Model file for the job. Use its own axes, mm. Face numbers are marked on the shaded views. A direction names the side the tool comes from. Round coordinates to 2 decimals unless told otherwise and drop trailing zeros. Order: outer loops, then holes, each group sorted by start corner. A loop starts at its lowest first (then second) coordinate and runs counter-clockwise, first axis right, second up. Notation, with made-up numbers: (58.25, 15) - (106.25, 15) arc R21 ccw to (106.25, 39) - close; hole circle Ø11 at (40.25, 70.25). An arc over 180 degrees is marked (long way). Write item = value, one per line.
```python
from build123d import *

# Parameters (mm, degrees)
F0_R          = 12.7
F1_DEPTH      = 76.2
F2_DEPTH      = 79.375
F2_DEPTH_BACK = 3.175
F4_DEPTH      = 50.8
F6_DEPTH      = 50.8


with BuildPart() as f1:
    # F0 (on Front) → F1 (new body)
    with BuildSketch(Plane.XZ):
        Circle(F0_R)
        Polygon((3.6661742094, 6.35), (5.499261351, 3.174999936), (7.3323484187, 0), (5.4992613448, -3.1749999467), (3.6661742094, -6.35), (0, -6.35), (-3.6661742094, -6.35), (-5.4992613166, -3.1749999956), (-7.3323484187, 0), (-5.4992612953, 3.1750000324), (-3.6661742094, 6.35), (0, 6.35), align=None, mode=Mode.SUBTRACT)
        with BuildLine():
            ThreePointArc((0, 6.35), (3.175000032, 5.4992612955), (5.499261351, 3.174999936))
            Line((5.499261351, 3.174999936), (3.6661742094, 6.35))
            Line((3.6661742094, 6.35), (0, 6.35))
        make_face()
        with BuildLine():
            ThreePointArc((5.499261351, 3.174999936), (6.1336290065, 1.6435009007), (6.35, 0))
            ThreePointArc((6.35, 0), (6.1336290049, -1.6435009067), (5.4992613448, -3.1749999467))
            Line((5.4992613448, -3.1749999467), (7.3323484187, 0))
            Line((7.3323484187, 0), (5.499261351, 3.174999936))
        make_face()
        with BuildLine():
            ThreePointArc((-5.4992612953, 3.1750000324), (-3.1749999838, 5.4992613234), (0, 6.35))
            Line((0, 6.35), (-3.6661742094, 6.35))
            Line((-3.6661742094, 6.35), (-5.4992612953, 3.1750000324))
        make_face()
        with BuildLine():
            ThreePointArc((-5.4992613166, -3.1749999956), (-6.35, 2.13e-08), (-5.4992612953, 3.1750000324))
            Line((-5.4992612953, 3.1750000324), (-7.3323484187, 0))
            Line((-7.3323484187, 0), (-5.4992613166, -3.1749999956))
        make_face()
        with BuildLine():
            Line((-3.6661742094, -6.35), (0, -6.35))
            ThreePointArc((0, -6.35), (-3.1750000022, -5.4992613128), (-5.4992613166, -3.1749999956))
            Line((-5.4992613166, -3.1749999956), (-3.6661742094, -6.35))
        make_face()
        with BuildLine():
            Line((3.6661742094, -6.35), (5.4992613448, -3.1749999467))
            ThreePointArc((5.4992613448, -3.1749999467), (3.1750000266, -5.4992612987), (0, -6.35))
            Line((0, -6.35), (3.6661742094, -6.35))
        make_face()
    extrude(amount=F1_DEPTH)

    # F0 (on Front) → F2 (join, two sides)
    with BuildSketch(Plane.XZ) as f2_sk:
        with BuildLine():
            ThreePointArc((5.4992613448, -3.1749999467), (6.1336290049, -1.6435009067), (6.35, 0))
            ThreePointArc((6.35, 0), (6.1336290065, 1.6435009007), (5.499261351, 3.174999936))
            ThreePointArc((5.499261351, 3.174999936), (3.175000032, 5.4992612955), (0, 6.35))
            ThreePointArc((0, 6.35), (-3.1749999838, 5.4992613234), (-5.4992612953, 3.1750000324))
            ThreePointArc((-5.4992612953, 3.1750000324), (-6.35, 2.13e-08), (-5.4992613166, -3.1749999956))
            ThreePointArc((-5.4992613166, -3.1749999956), (-3.1750000022, -5.4992613128), (0, -6.35))
            ThreePointArc((0, -6.35), (3.1750000266, -5.4992612987), (5.4992613448, -3.1749999467))
        make_face()
    extrude(amount=F2_DEPTH)
    extrude(f2_sk.sketch, amount=-F2_DEPTH_BACK)

    # F3 (on face) → F4 (join)
    with BuildSketch(Plane(origin=(0, 3.175, 0), x_dir=(-1, 0, 0), z_dir=(0, 1, 0))):
        Polygon((6.35, -3.6661742094), (6.35, 3.6661742094), (0, 7.3323484187), (-6.35, 3.6661742094), (-6.35, -3.6661742094), (0, -7.3323484187), align=None)
    extrude(amount=F4_DEPTH)

    # F5 (on face) → F6 (join)
    with BuildSketch(Plane.XZ.offset(79.375)):
        Polygon((-6.35, 3.6661742094), (-6.35, -3.6661742094), (0, -7.3323484187), (6.35, -3.6661742094), (6.35, 3.6661742094), (0, 7.3323484187), align=None)
    extrude(amount=F6_DEPTH)


solid = f1.part
```
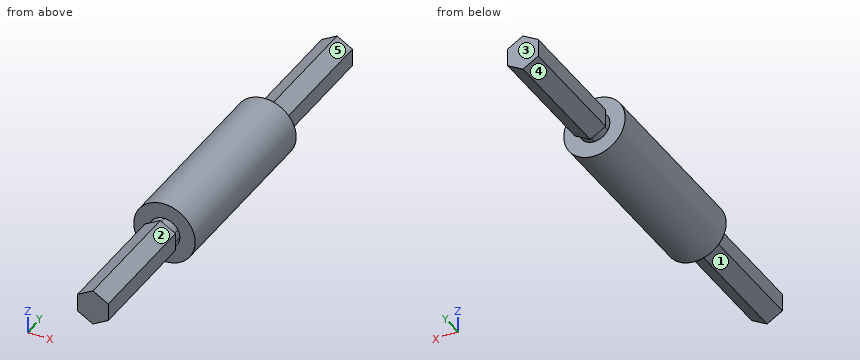
1) 3-axis set-ups, long thin cutter, end or side, ignore diameter. For the marked faces 1, 2, 3, 4 and 5: which of +Z, -Z, +X, -X, +Y, -Y reach the whole face in a straight line?
Conclusion:
face_1 = -Z, -X, -Y
face_2 = +Z, +X, -Y
face_3 = +Z, -Z, +X, -X, +Y
face_4 = -Z, -X, +Y
face_5 = +Z, +X, +Y
2) Cut at A-A (y = -116). Write the cut outline in (x, z), and give its area (3 significant figures).
Conclusion:
outline = (-6.35, -3.67) - (0, -7.33) - (6.35, -3.67) - (6.35, 3.67) - (0, 7.33) - (-6.35, 3.67) - close
area = 140 mm^2
3) Wall check: line 1 along X through (y, z) = (-14.5, 11); line 2 along Y through (x, z) = (7.25, 5.25); line 3 along Z through (x, y) = (0, -81.5). Give the ranges that are in metal, low to high.
Conclusion:
line_1 = -6.35 to 6.35
line_2 = -76.2 to 0
line_3 = -7.33 to 7.33
4) Cut at C-C (x = -9.5). Write the cut outline in (y, z).
Conclusion:
outline = (-76.2, -8.43) - (0, -8.43) - (0, 8.43) - (-76.2, 8.43) - close
5) Cut at B-B (x = 10.25). Write the cut outline in (y, z), and give its area (3 significant figures).
Conclusion:
outline = (-76.2, -7.5) - (0, -7.5) - (0, 7.5) - (-76.2, 7.5) - close
area = 1,140 mm^2
6) Flat gauge pins, fed straight in: pin 1 Ø8 at (y, z) = (30, -0.5) entering from +X; pin 2 Ø6 at (x, y) = (-5.5, -51.5) entering from +Z; pin 3 Ø6 at (y, z) = (-69.5, 4.5) entering from -X; pin 4 Ø1.5 at (x, y) = (8.5, -102.5) entering from +Z. Where does each tip first touch, or does it go through?
Conclusion:
pin_1 = 6.35
pin_2 = 12.45
pin_3 = -12.61
pin_4 = through
